Model file for the job. Use its own axes, mm. Face numbers are marked on the shaded views. A direction names the side the tool comes from. Round coordinates to 2 decimals unless told otherwise and drop trailing zeros. Order: outer loops, then holes, each group sorted by start corner. A loop starts at its lowest first (then second) coordinate and runs counter-clockwise, first axis right, second up. Notation, with made-up numbers: (55.25, -11) - (72.25, -11) arc R20 ccw to (72.25, 11) - close; hole circle Ø8 at (12.25, 50.5). An arc over 180 degrees is marked (long way). Put each result on its own line as item: value. Start each with the question number.
Item 1: Saw through at B-B on x = 12.7. List the corners of the cut face in (y, z).
Item 2: Which spindle directions (+Z, -Z, +X, -X, +Y, -Y) get a long thin tool onto all of the face, cutting with end or side? Do the marked faces 1 and 2. Say none if no direction does.
Item 3: Saw through at D-D on x = 19.5. List the corners of the cut face in (y, z).
Item 4: Probe probe 1 along X at (y, z) = (133.35, -0.55); probe 2 along Y at (x, z) = (6.35, -1.1); probe 3 along X at (y, z) = (81, -21). List the from-to ranges inside material, lowest first.
Item 5: Pin check, flat tips, straight feed: pin 1 Ø4 at (x, y) = (6.35, 133.35) entering from +Z; pin 2 Ø4 at (x, y) = (12.7, 139.7) entering from -Z; pin 3 Ø5 at (x, z) = (4.5, -39.5) entering from -Y. Stop position of each tip, or through.
Item 6: Mould opens along X. For the marked faces 3, 4 and 5 say: pulls with the +X half, pulls with the -X half, needs draft (parallel to the pull), parting line crosses it, or undercut.
Item 7: Saw through at C-C on y = 75. List the corners of the cut face in (x, z), plus the area to 3 significant figures.
Item 8: Saw through at A-A on z = -12.7. List the corners of the cut face in (x, y), plus the area to 3 significant figures.
```python
from build123d import *

# Parameters (mm, degrees)
BOSS_EXTRUDE1_DEPTH = 177.8
SKETCH2_R           = 10.16
SKETCH2_R_2         = 3.429
CUT_EXTRUDE1_DEPTH  = 12.7
SKETCH2_3_R         = 3.429
CUT_EXTRUDE2_DEPTH  = 26.4
SKETCH3_R           = 3.429
CUT_EXTRUDE3_DEPTH  = 2.54
SKETCH4_R           = 3.429
CUT_EXTRUDE4_DEPTH  = 2.54


with BuildPart() as part:
    # Sketch1 → Boss-Extrude1 (new body)
    with BuildSketch(Plane(origin=(0, 0, 0), x_dir=(1, 0, 0), z_dir=(0, 1, 0))):
        with BuildLine():
            Line((0.254, 50.8), (25.146, 50.8))
            ThreePointArc((25.146, 50.8), (25.325605122, 50.725605122), (25.4, 50.546))
            Line((25.4, 50.546), (25.4, 0.254))
            ThreePointArc((25.4, 0.254), (25.325605122, 0.074394878), (25.146, 0))
            Line((25.146, 0), (0.254, 0))
            ThreePointArc((0.254, 0), (0.074394878, 0.074394878), (0, 0.254))
            Line((0, 0.254), (0, 50.546))
            ThreePointArc((0, 50.546), (0.074394878, 50.725605122), (0.254, 50.8))
        make_face()
        with BuildLine():
            Line((1.5875, 3.1115), (1.5875, 47.6885))
            ThreePointArc((1.5875, 47.6885), (2.033869265, 48.766130735), (3.1115, 49.2125))
            Line((3.1115, 49.2125), (22.2885, 49.2125))
            ThreePointArc((22.2885, 49.2125), (23.366130735, 48.766130735), (23.8125, 47.6885))
            Line((23.8125, 47.6885), (23.8125, 3.1115))
            ThreePointArc((23.8125, 3.1115), (23.366130735, 2.033869265), (22.2885, 1.5875))
            Line((22.2885, 1.5875), (3.1115, 1.5875))
            ThreePointArc((3.1115, 1.5875), (2.033869265, 2.033869265), (1.5875, 3.1115))
        make_face(mode=Mode.SUBTRACT)
    extrude(amount=BOSS_EXTRUDE1_DEPTH)

    # Sketch2 → Cut-Extrude1 (cut)
    with BuildSketch(Plane.ZY):
        with Locations((-25.4, 12.192)):
            Circle(SKETCH2_R)
        with Locations((-25.4, 12.192)):
            Circle(SKETCH2_R_2, mode=Mode.SUBTRACT)
        with Locations((-25.4, 62.992)):
            Circle(SKETCH2_R)
        with Locations((-25.4, 62.992)):
            Circle(SKETCH2_R_2, mode=Mode.SUBTRACT)
        with Locations((-38.1, 165.1)):
            Circle(SKETCH2_R_2)
        with Locations((-25.4, 165.1)):
            Circle(SKETCH2_R_2)
        with Locations((-12.7, 165.1)):
            Circle(SKETCH2_R_2)
        with Locations((-25.4, 133.35)):
            Circle(SKETCH2_R_2)
        with Locations((-12.7, 133.35)):
            Circle(SKETCH2_R_2)
        with Locations((-25.4, 101.6)):
            Circle(SKETCH2_R_2)
        with Locations((-12.7, 101.6)):
            Circle(SKETCH2_R_2)
        with Locations((-38.1, 133.35)):
            Circle(SKETCH2_R_2)
        with Locations((-38.1, 101.6)):
            Circle(SKETCH2_R_2)
    extrude(amount=-CUT_EXTRUDE1_DEPTH, mode=Mode.SUBTRACT)

    # Sketch2_3 → Cut-Extrude2 (cut, through all)
    with BuildSketch(Plane.ZY):
        with Locations((-25.4, 12.192)):
            Circle(SKETCH2_3_R)
        with Locations((-25.4, 62.992)):
            Circle(SKETCH2_3_R)
    extrude(amount=-CUT_EXTRUDE2_DEPTH, mode=Mode.SUBTRACT)

    # Sketch3 → Cut-Extrude3 (cut)
    with BuildSketch(Plane.XY):
        with Locations((19.05, 165.1)):
            Circle(SKETCH3_R)
        with Locations((6.35, 165.1)):
            Circle(SKETCH3_R)
        with Locations((6.35, 133.35)):
            Circle(SKETCH3_R)
        with Locations((6.35, 101.6)):
            Circle(SKETCH3_R)
        with Locations((19.05, 133.35)):
            Circle(SKETCH3_R)
        with Locations((19.05, 101.6)):
            Circle(SKETCH3_R)
    extrude(amount=-CUT_EXTRUDE3_DEPTH, mode=Mode.SUBTRACT)

    # Sketch4 → Cut-Extrude4 (cut)
    with BuildSketch(Plane(origin=(0, 0, -50.8), x_dir=(-1, 0, 0), z_dir=(0, 0, -1))):
        with Locations((-12.7, 165.1)):
            Circle(SKETCH4_R)
        with Locations((-12.7, 139.7)):
            Circle(SKETCH4_R)
        with Locations((-12.7, 127)):
            Circle(SKETCH4_R)
        with Locations((-12.7, 101.6)):
            Circle(SKETCH4_R)
    extrude(amount=-CUT_EXTRUDE4_DEPTH, mode=Mode.SUBTRACT)


solid = part.part
```
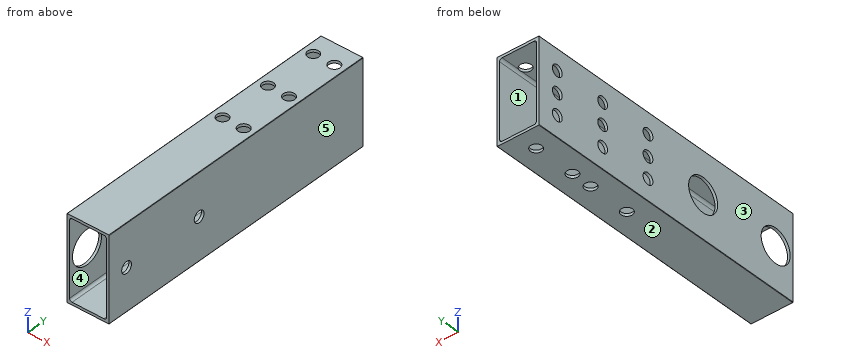
Results found:
1. outline: (0, -50.8) - (98.17, -50.8) - (98.17, -49.21) - (0, -49.21) - close; (0, -1.59) - (177.8, -1.59) - (177.8, 0) - (0, 0) - close; (105.03, -50.8) - (123.57, -50.8) - (123.57, -49.21) - (105.03, -49.21) - close; (130.43, -50.8) - (136.27, -50.8) - (136.27, -49.21) - (130.43, -49.21) - close; (143.13, -50.8) - (161.67, -50.8) - (161.67, -49.21) - (143.13, -49.21) - close; (168.53, -50.8) - (177.8, -50.8) - (177.8, -49.21) - (168.53, -49.21) - close
2. face 1: +Y, -Y
2. face 2: -Z, +X, -X, +Y, -Y
3. outline: (0, -50.8) - (177.8, -50.8) - (177.8, -49.21) - (0, -49.21) - close; (0, -1.59) - (98.2, -1.59) - (98.2, 0) - (0, 0) - close; (105, -1.59) - (129.95, -1.59) - (129.95, 0) - (105, 0) - close; (136.75, -1.59) - (161.7, -1.59) - (161.7, 0) - (136.75, 0) - close; (168.5, -1.59) - (177.8, -1.59) - (177.8, 0) - (168.5, 0) - close
4. probe 1: x = 0 to 2.92, 9.78 to 15.62, 22.48 to 25.4
4. probe 2: y = 0 to 98.17, 105.03 to 129.92, 136.78 to 161.67, 168.53 to 177.8
4. probe 3: x = 0 to 1.59, 23.81 to 25.4
5. pin 1: stops at z = -49.21
5. pin 2: stops at z = -1.59
5. pin 3: passes through
6. face 3: pulls with the -X half
6. face 4: undercut
6. face 5: pulls with the +X half
7. outline: (0, -50.55) arc R0.25 ccw to (0.25, -50.8) - (25.15, -50.8) arc R0.25 ccw to (25.4, -50.55) - (25.4, -0.25) arc R0.25 ccw to (25.15, 0) - (0.25, 0) arc R0.25 ccw to (0, -0.25) - close; hole (1.59, -47.69) arc R1.52 ccw to (3.11, -49.21) - (22.29, -49.21) arc R1.52 ccw to (23.81, -47.69) - (23.81, -3.11) arc R1.52 ccw to (22.29, -1.59) - (3.11, -1.59) arc R1.52 ccw to (1.59, -3.11) - close
7. area: 234 mm²
8. outline: (0, 0) - (1.59, 0) - (1.59, 98.17) - (0, 98.17) - close; (0, 105.03) - (1.59, 105.03) - (1.59, 129.92) - (0, 129.92) - close; (0, 136.78) - (1.59, 136.78) - (1.59, 161.67) - (0, 161.67) - close; (0, 168.53) - (1.59, 168.53) - (1.59, 177.8) - (0, 177.8) - close; (23.81, 0) - (25.4, 0) - (25.4, 177.8) - (23.81, 177.8) - close
8. area: 532 mm²
